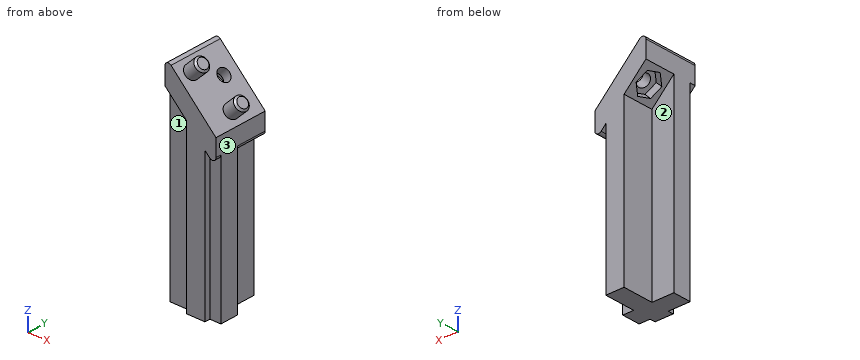
from build123d import *

# Parameters (mm, degrees)
PAD001_DEPTH         = 25
PAD001_DEPTH_BACK    = 26
POCKET004_DEPTH      = 7.501
POCKET004_DEPTH_BACK = 7.501
PAD002_DEPTH         = 15
POCKET005_DEPTH      = 2.15
SKETCH011_R          = 1.7
HOLE001_DEPTH        = 12.7504949366
SKETCH012_R          = 1.9
PAD003_DEPTH         = 4.5
CHAMFER_SIZE         = 0.5
FILLET001_R          = 1


with BuildPart() as part:
    # Sketch007 → Pad001 (new body, two sides)
    with BuildSketch(Plane.XY) as pad001_sk:
        Polygon((-7, -6), (-1, -6), (-1, -7.5), (4, -7.5), (4, -6), (7, -6), (7, -1), (4, -1), (4, 7.5), (-1, 7.5), (-1, -1), (-7, -1), align=None)
    extrude(amount=PAD001_DEPTH)
    extrude(pad001_sk.sketch, amount=-PAD001_DEPTH_BACK)

    # Sketch008 → Pocket004 (cut, two sides)
    with BuildSketch(Plane.XZ) as pocket004_sk:
        Polygon((-7, 25), (7, 11), (7, 25), align=None)
    extrude(amount=-POCKET004_DEPTH, mode=Mode.SUBTRACT)
    extrude(pocket004_sk.sketch, amount=POCKET004_DEPTH_BACK, mode=Mode.SUBTRACT)

    # Sketch009 (on Face8 of Pocket004) → Pad002 (join)
    with BuildSketch(Plane.XZ.offset(7.5)):
        Polygon((-7, 25), (7, 11), (7, 18.0710678119), (-7, 32.0710678119), align=None)
    extrude(amount=-PAD002_DEPTH)

    # Sketch010 (on Face12 of Pad002) → Pocket005 (cut)
    with BuildSketch(Plane(origin=(9, 0, 9), x_dir=(0.7071067812, 0, -0.7071067812), z_dir=(-0.7071067812, 0, -0.7071067812))):
        Polygon((-21.5619467058, -2.3333103769), (-20.6952570827, -5.5678400847), (-17.4607273749, -6.4345297078), (-15.0928872902, -4.0666896231), (-15.9595769133, -0.8321599153), (-19.1941066211, 0.0345297078), align=None)
    extrude(amount=-POCKET005_DEPTH, mode=Mode.SUBTRACT)

    # Sketch011 (on Face29 of Pocket005) → Hole001 (cut, through all)
    with BuildSketch(Plane(origin=(10.5202795796, 0, 10.5202795796), x_dir=(0, -1, 0), z_dir=(-0.7071067812, 0, -0.7071067812))):
        with Locations((-3.2, 18.327416998)):
            Circle(SKETCH011_R)
    extrude(amount=-HOLE001_DEPTH, mode=Mode.SUBTRACT)

    # Sketch012 (on Face9 of Hole001) → Pad003 (join)
    with BuildSketch(Plane(origin=(12.5355339059, 0, 12.5355339059), x_dir=(0.7071067812, 0, -0.7071067812), z_dir=(0.7071067812, 0, 0.7071067812))):
        with Locations((-22.027416998, -3.8)):
            Circle(SKETCH012_R)
        with Locations((-11.127416998, -0.3)):
            Circle(SKETCH012_R)
    extrude(amount=PAD003_DEPTH)

    # Chamfer
    chamfer_edges = [part.edges().sort_by_distance(p)[0] for p in [
        (-1.201724, -3.8, 32.636753),
        (6.50574, -0.3, 24.929289),
    ]]
    chamfer(chamfer_edges, length=CHAMFER_SIZE)

    # Fillet001
    fillet001_edges = [part.edges().sort_by_distance(p)[0] for p in [
        (-7, 0, 32.071068),
        (7, 3.25, 11),
        (7, -6.75, 11),
    ]]
    fillet(fillet001_edges, radius=FILLET001_R)


with BuildPart() as part_1:
    # Body001 placement: moved
    add(part.part.moved(Location((0, 0, 33))))


solid = part_1.part
Verification items for the finished model (mm, model axes). Face numbers are marked on the shaded views. A direction names the side the tool comes from. Coordinates: 2 decimals unless noted, no trailing zeros. Loops run counter-clockwise (first coordinate to the right, second up) from the corner with the lowest first, then second, coordinate; pieces in that order, holes last. Notation, with made-up numbers: M 47.25,63.25 L 79.25,63.25 A7 cw 79.25,71.25 Z; hole C -37,60.25 d6. An arc over 180 degrees is marked long. One line per item, written item: value.
1. Section check A-A on z = 47.5. Record the cut outline in (x, y), plus the area to 3 significant figures.
Answers follow:
outline: M -7,-6 L -1,-6 L -1,-7.5 L 7,-7.5 L 7,7.5 L -1,7.5 L -1,-1 L -7,-1 Z
area: 150 mm^2
2. Gauge pin test, flat ends, axial feed: P1, Ø1, axis at y = -5, z = 27.5, coming from the +X side; P2, Ø4, axis at y = 3.5, z = 39, coming from the -X side; P3, Ø1.8, axis at x = -4.5, z = 33.5, coming from the +Y side. Record the tip position at first contact, or that the pin passes through.
Answers follow:
P1: x = 7
P2: x = -1
P3: y = -1
3. Section check B-B on z = 35.5. Record the cut outline in (x, y), plus the area to 3 significant figures.
Answers follow:
outline: M -7,-6 L -1,-6 L -1,-7.5 L 4,-7.5 L 4,-6 L 7,-6 L 7,-1 L 4,-1 L 4,7.5 L -1,7.5 L -1,-1 L -7,-1 Z
area: 120 mm^2
4. Material ranges on line 1 along X through (y, z) = (-2.5, 48); line 2 along Y through (x, z) = (-3.5, 32); line 3 along X through (y, z) = (7.25, 28), recorded low to high. Write a range as from..to.
Answers follow:
line 1: -7..7
line 2: -6..-1
line 3: -1..4
5. Set-up check for the marked faces 1, 2 and 3: record each of +Z, -Z, +X, -X, +Y, -Y from which the full face is reachable in a straight line by a thin tool's end or side.
Answers follow:
face 1: -Z, -X, -Y
face 2: -Z, -X, +Y
face 3: -Z, +X, +Y, -Y
